Input: part model. Units: mm. Frame: model coordinates. Face numbers are marked on the shaded views. A direction names the side the tool comes from. Round coordinates to 2 decimals unless told otherwise and drop trailing zeros. Loops run counter-clockwise (first coordinate to the right, second up) from the corner with the lowest first, then second, coordinate; pieces in that order, holes last. Notation, with made-up numbers: (63.5, 33.5) -> (84.5, 33.5) arc R25 cw to (84.5, 54.5) -> close; hole circle Ø2 at (52, -4.75). An arc over 180 degrees is marked (long way). One line per question, with ' | ' between items. Start each with the question number.
Q1. Cut plane C-C on y = -4.5. Return loops of the section in (x, z), and give its area (3 significant figures).
Q2. Access query for the marked faces 5, 6, 7 and 8. Directions: +Z, -Z, +X, -X, +Y, -Y. A direction counts if a zero-diameter tool reaches every point of the face in a straight line with its end or side. Return the directions, or none.
Q3. Material intervals for L1, parallel to X at y = -4.25, z = -3.5; L2, parallel to Z at x = -1.5, y = -3.25; L3, parallel to X at y = -6.25, z = -9.5, sorted ascending.
Q4. Cut plane B-B on z = 0. Return loops of the section in (x, y), and give its area (3 significant figures).
Q5. Mould query, pull axis Z, two halves, no side actions, for the marked faces 1, 2, 3 and 4. Classes: pulls with the +Z half, pulls with the -Z half, needs draft (parallel to the pull), parting line crosses it, or undercut.
Q6. Contact query for flat-ended pins moving along their axis: P1, Ø1.9, axis at y = -2.5, z = -16.5, coming from the -X side; P2, Ø4, axis at y = -1, z = 3, coming from the +X side; P3, Ø6, axis at x = -6, z = 7.5, coming from the -Y side; P4, Ø3.5, axis at x = 3, y = -4, coming from the -Z side. Output: stop coordinate, or through.
Q7. Cut plane D-D on z = 10.5. Return loops of the section in (x, y).
Q8. Cut plane A-A on x = -5. Return loops of the section in (y, z).
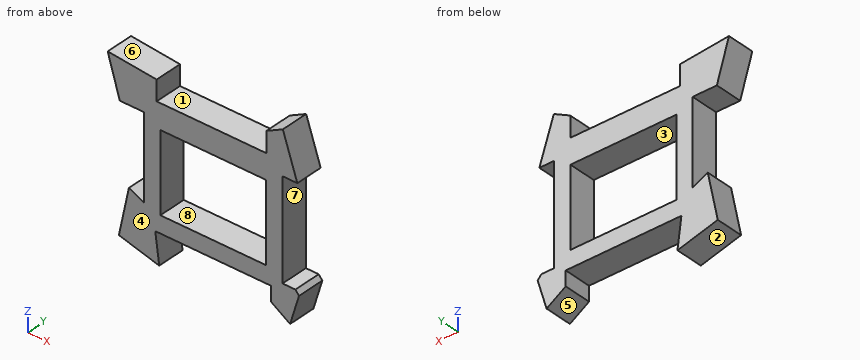
from build123d import *

# Parameters (mm, degrees)
F1_DEPTH = 7


with BuildPart() as f1:
    # F0 (on Front) → F1 (new body)
    with BuildSketch(Plane.XZ):
        Polygon((13.480433, 15.230299), (0, 15.230299), (-14.4018, 15.230299), (-14.4018, 20.327233), (-26.8478, 21.512566), (-23.765933, 11.318699), (-17.6022, 11.318699), (-17.6022, -9.879558), (-21.452855, -8.042291), (-24.001321, -20.191958), (-13.748187, -22.858959), (-14.755721, -15.232768), (0, -15.232768), (14.653853, -15.232768), (14.653853, -18.953877), (19.515166, -22.05506), (21.778191, -14.511641), (20.856217, -13.422038), (17.6022, -13.422038), (17.6022, 11.638863), (21.359112, 11.638863), (17.67122, 22.618724), (13.480433, 20.439515), align=None)
        Polygon((-13.453534, 8.948033), (0, 8.948033), (13.453534, 8.948033), (13.453534, -10.965568), (0, -10.965568), (-13.453534, -10.965568), align=None, mode=Mode.SUBTRACT)
    extrude(amount=F1_DEPTH)


solid = f1.part
Results:
1) outline: (-26.85, 21.51) -> (-23.77, 11.32) -> (-17.6, 11.32) -> (-17.6, -9.88) -> (-21.45, -8.04) -> (-24, -20.19) -> (-13.75, -22.86) -> (-14.76, -15.23) -> (14.65, -15.23) -> (14.65, -18.95) -> (19.52, -22.06) -> (21.78, -14.51) -> (20.86, -13.42) -> (17.6, -13.42) -> (17.6, 11.64) -> (21.36, 11.64) -> (17.67, 22.62) -> (13.48, 20.44) -> (13.48, 15.23) -> (-14.4, 15.23) -> (-14.4, 20.33) -> close; hole (-13.45, -10.97) -> (13.45, -10.97) -> (13.45, 8.95) -> (-13.45, 8.95) -> close | area: 802 mm^2
2) face 5: -Z, +Y, -Y | face 6: +Z, +Y, -Y | face 7: +X, +Y, -Y | face 8: +Y, -Y
3) L1: -17.6 to -13.45, 13.45 to 17.6 | L2: -15.23 to -10.97, 8.95 to 15.23 | L3: -21.76 to -18.4, -17.6 to -13.45, 13.45 to 17.6
4) outline: (-17.6, -7) -> (-13.45, -7) -> (-13.45, 0) -> (-17.6, 0) -> close; (13.45, -7) -> (17.6, -7) -> (17.6, 0) -> (13.45, 0) -> close | area: 58.1 mm^2
5) face 1: pulls with the +Z half | face 2: pulls with the -Z half | face 3: undercut | face 4: needs draft
6) P1: x = -23.43 | P2: x = 17.6 | P3: y = -7 | P4: z = -15.23
7) outline: (-17.6, -7) -> (17.6, -7) -> (17.6, 0) -> (-17.6, 0) -> close
8) outline: (-7, -15.23) -> (0, -15.23) -> (0, -10.97) -> (-7, -10.97) -> close; (-7, 8.95) -> (0, 8.95) -> (0, 15.23) -> (-7, 15.23) -> close
